Input: part model. Units: mm. Frame: model coordinates. Round coordinates to 2 decimals unless told otherwise and drop trailing zeros.
(1) Line query: line 1 (Y direction, x = -25, z = 508); line 2 (X direction, y = -12, z = 1079.5); line 3 (X direction, y = -9, z = 1698.5). Output: solid intervals per line, ascending.
(2) Cut plane A-A, the plane z = 889.5. Give the number of separate pieces and of enclosed holes in the cut face, and give its area (3 significant figures).
(3) First-contact query: pin 1 Ø3 at (y, z) = (-16, 1419.5) entering from -X. Flat tip, straight axial feed; report the tip coordinate or a pass-through.
from build123d import *

# Parameters (mm, degrees)
F0_R     = 3
F0_R_2   = 2.5
F1_DEPTH = 1890
F2_R     = 2
F3_R     = 7


# Not quite as in the source:
# - a feature names something its author has since deleted; it is built from what else it names


with BuildPart() as f1:
    # F0 (on Top) → F1 (new body)
    with BuildSketch(Plane.XY):
        with BuildLine():
            Line((18.15, -30), (30, -30))
            Line((30, -30), (30, -18.15))
            Line((30, -18.15), (27.5, -18.15))
            Line((27.5, -18.15), (27.5, -20.15))
            Line((27.5, -20.15), (21.5477069044, -20.15))
            ThreePointArc((21.5477069044, -20.15), (19.5, -15), (21.5477069044, -9.85))
            Line((21.5477069044, -9.85), (27.5, -9.85))
            Line((27.5, -9.85), (27.5, -11.85))
            Line((27.5, -11.85), (30, -11.85))
            Line((30, -11.85), (30, 11.85))
            Line((30, 11.85), (27.5, 11.85))
            Line((27.5, 11.85), (27.5, 9.85))
            Line((27.5, 9.85), (21.5477069044, 9.85))
            ThreePointArc((21.5477069044, 9.85), (19.5, 15), (21.5477069044, 20.15))
            Line((21.5477069044, 20.15), (27.5, 20.15))
            Line((27.5, 20.15), (27.5, 18.15))
            Line((27.5, 18.15), (30, 18.15))
            Line((30, 18.15), (30, 30))
            Line((30, 30), (18.15, 30))
            Line((18.15, 30), (18.15, 27.5))
            Line((18.15, 27.5), (20.15, 27.5))
            Line((20.15, 27.5), (20.15, 21.5477069044))
            ThreePointArc((20.15, 21.5477069044), (15, 19.5), (9.85, 21.5477069044))
            Line((9.85, 21.5477069044), (9.85, 27.5))
            Line((9.85, 27.5), (11.85, 27.5))
            Line((11.85, 27.5), (11.85, 30))
            Line((11.85, 30), (-11.85, 30))
            Line((-11.85, 30), (-11.85, 27.5))
            Line((-11.85, 27.5), (-9.85, 27.5))
            Line((-9.85, 27.5), (-9.85, 21.5477069044))
            ThreePointArc((-9.85, 21.5477069044), (-15, 19.5), (-20.15, 21.5477069044))
            Line((-20.15, 21.5477069044), (-20.15, 27.5))
            Line((-20.15, 27.5), (-18.15, 27.5))
            Line((-18.15, 27.5), (-18.15, 30))
            Line((-18.15, 30), (-30, 30))
            Line((-30, 30), (-30, 18.15))
            Line((-30, 18.15), (-27.5, 18.15))
            Line((-27.5, 18.15), (-27.5, 20.15))
            Line((-27.5, 20.15), (-21.5477069044, 20.15))
            ThreePointArc((-21.5477069044, 20.15), (-19.5, 15), (-21.5477069044, 9.85))
            Line((-21.5477069044, 9.85), (-27.5, 9.85))
            Line((-27.5, 9.85), (-27.5, 11.85))
            Line((-27.5, 11.85), (-30, 11.85))
            Line((-30, 11.85), (-30, -11.85))
            Line((-30, -11.85), (-27.5, -11.85))
            Line((-27.5, -11.85), (-27.5, -9.85))
            Line((-27.5, -9.85), (-21.5477069044, -9.85))
            ThreePointArc((-21.5477069044, -9.85), (-19.5, -15), (-21.5477069044, -20.15))
            Line((-21.5477069044, -20.15), (-27.5, -20.15))
            Line((-27.5, -20.15), (-27.5, -18.15))
            Line((-27.5, -18.15), (-30, -18.15))
            Line((-30, -18.15), (-30, -30))
            Line((-30, -30), (-18.15, -30))
            Line((-18.15, -30), (-18.15, -27.5))
            Line((-18.15, -27.5), (-20.15, -27.5))
            Line((-20.15, -27.5), (-20.15, -21.5477069044))
            ThreePointArc((-20.15, -21.5477069044), (-15, -19.5), (-9.85, -21.5477069044))
            Line((-9.85, -21.5477069044), (-9.85, -27.5))
            Line((-9.85, -27.5), (-11.85, -27.5))
            Line((-11.85, -27.5), (-11.85, -30))
            Line((-11.85, -30), (11.85, -30))
            Line((11.85, -30), (11.85, -27.5))
            Line((11.85, -27.5), (9.85, -27.5))
            Line((9.85, -27.5), (9.85, -21.5477069044))
            ThreePointArc((9.85, -21.5477069044), (15, -19.5), (20.15, -21.5477069044))
            Line((20.15, -21.5477069044), (20.15, -27.5))
            Line((20.15, -27.5), (18.15, -27.5))
            Line((18.15, -27.5), (18.15, -30))
        make_face()
        with Locations((-25, -25)):
            Circle(F0_R, mode=Mode.SUBTRACT)
        with Locations((-15, -15)):
            Circle(F0_R_2, mode=Mode.SUBTRACT)
        with Locations((25, -25)):
            Circle(F0_R, mode=Mode.SUBTRACT)
        with Locations((15, -15)):
            Circle(F0_R_2, mode=Mode.SUBTRACT)
        with Locations((-25, 25)):
            Circle(F0_R, mode=Mode.SUBTRACT)
        with Locations((-15, 15)):
            Circle(F0_R_2, mode=Mode.SUBTRACT)
        Polygon((-7, 22), (-7, 27.5), (0, 27.5), (7, 27.5), (7, 22), (10, 16), (10, 10), (16, 10), (22, 7), (27.5, 7), (27.5, 0), (27.5, -7), (22, -7), (16, -10), (10, -10), (10, -16), (7, -22), (7, -27.5), (0, -27.5), (-7, -27.5), (-7, -22), (-10, -16), (-10, -10), (-16, -10), (-22, -7), (-27.5, -7), (-27.5, 0), (-27.5, 7), (-22, 7), (-16, 10), (-10, 10), (-10, 16), align=None, mode=Mode.SUBTRACT)
        with Locations((15, 15)):
            Circle(F0_R_2, mode=Mode.SUBTRACT)
        with Locations((25, 25)):
            Circle(F0_R, mode=Mode.SUBTRACT)
    extrude(amount=F1_DEPTH)

    # F2
    f2_edges = [f1.edges().sort_by_distance(p)[0] for p in [
        (-7, 27.5, 945),
        (7, 27.5, 945),
    ]]
    fillet(f2_edges, radius=F2_R)

    # F3
    f3_edges = [f1.edges().sort_by_distance(p)[0] for p in [
        (-10, 16, 945),
        (10, 16, 945),
    ]]
    fillet(f3_edges, radius=F3_R)


solid = f1.part
Reported:
1. line 1: y = -30 to -28, -22 to -20.15, -9.85 to -7, 7 to 9.85, 20.15 to 22, 28 to 30
1. line 2: x = -20.13 to -10, 10 to 20.13
1. line 3: x = -30 to -18, 18 to 30
2. separate pieces: 1
2. enclosed holes: 9
2. area: 1,080 mm2
3. pin 1: stops at x = -19.93
